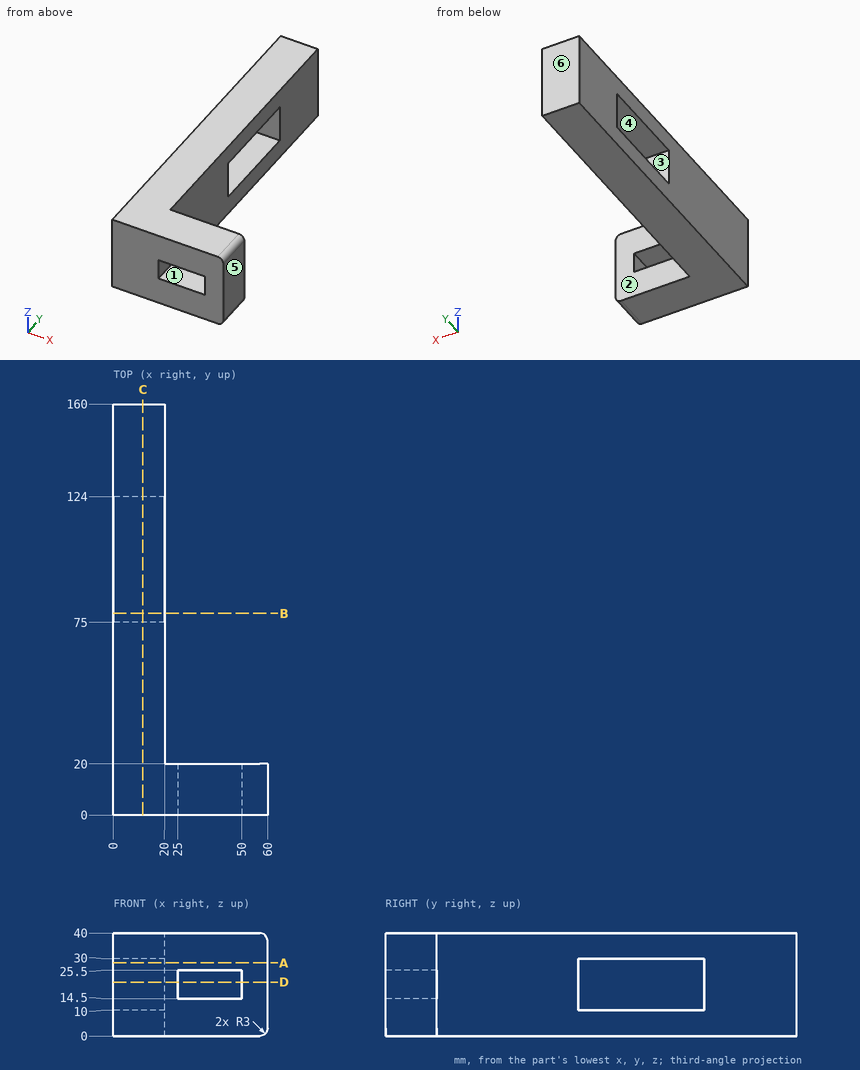
The drawing under review shows one solid part. Ordinate dimensions are in mm from its lowest x, y, z. A direction names the side the tool comes from. Give positions to 0.01 mm unless a question says otherwise; leave off trailing zeros. Write each loop counter-clockwise with the first axis right and the second up, starting at its lowest first coordinate (ties: lowest second). Pieces come first, ordered by that corner, then holes. Notation, with made-up numbers: (-7.5, -32.75) -> (8.5, -32.75) arc R22 ccw to (8.5, -0.75) -> close; hole circle Ø9 at (-33, -26). An arc over 180 degrees is marked (long way). Answer in a Markdown table with one row per item.
(1) Consider section B-B (y = 78.5). State the section outline as (x, z) points.
Results:
| item | result |
|---|---|
| outline | (0, 0) -> (20, 0) -> (20, 10) -> (0, 10) -> close; (0, 30) -> (20, 30) -> (20, 40) -> (0, 40) -> close |
(2) Consider section D-D (z = 21). State the section outline as (x, y) points, then the cut area to 3 significant figures.
Results:
| item | result |
|---|---|
| outline | (0, 0) -> (25, 0) -> (25, 20) -> (20, 20) -> (20, 75) -> (0, 75) -> close; (0, 124) -> (20, 124) -> (20, 160) -> (0, 160) -> close; (50, 0) -> (60, 0) -> (60, 20) -> (50, 20) -> close |
| area | 2,520 mm2 |
(3) To check wall thickness, follow probe 1 along Z at (x, y) = (6.5, 97.5); probe 2 along Y at (x, z) = (13, 13); probe 3 along X at (y, z) = (65.5, 10). State the ranges of each line that lie inside material, in increasing order.
Results:
| item | result |
|---|---|
| probe 1 | 0 to 10, 30 to 40 |
| probe 2 | 0 to 75, 124 to 160 |
| probe 3 | 0 to 20 |
(4) Clearance check with flat-ended pins moving along their axes: pin 1 (2 mm diameter, centred on y = 95, z = 33, fed in from +X); pin 2 (20 mm diameter, centred on x = 37, z = 22, fed in from +Y). State where each tip first meets the part, or that it passes through.
Results:
| item | result |
|---|---|
| pin 1 | x = 20 |
| pin 2 | y = 20 |
(5) Mouldability with a two-part tool opening along Y and no side actions: class the marked faces 4, 5 and 6 as +Y half, -Y half, draft (parallel to the pull), parting line (faces both ways), or undercut.
Results:
| item | result |
|---|---|
| face 4 | undercut |
| face 5 | draft |
| face 6 | +Y half |
(6) For the marked faces 1, 2 and 3, list the 3-axis set-ups (+Z, -Z, +X, -X, +Y, -Y) from which the entire face can be reached by the end or side of a thin tool; tool diameter is ignored.
Results:
| item | result |
|---|---|
| face 1 | +Y, -Y |
| face 2 | +Z, -Z, +X, +Y |
| face 3 | +X, -X |
(7) Consider section A-A (z = 28.5). State the section outline as (x, y) points.
Results:
| item | result |
|---|---|
| outline | (0, 0) -> (60, 0) -> (60, 20) -> (20, 20) -> (20, 75) -> (0, 75) -> close; (0, 124) -> (20, 124) -> (20, 160) -> (0, 160) -> close |
(8) Consider section C-C (x = 11.5). State the section outline as (y, z) points, then the cut area to 3 significant figures.
Results:
| item | result |
|---|---|
| outline | (0, 0) -> (160, 0) -> (160, 40) -> (0, 40) -> close; hole (75, 10) -> (124, 10) -> (124, 30) -> (75, 30) -> close |
| area | 5,420 mm2 |
